The listing builds one solid part. Answer for the finished solid, in the listing's coordinates (mm). A direction names the side the tool comes from. Give positions to 0.01 mm unless a question says otherwise; leave off trailing zeros. Order: outer loops, then holes, each group sorted by start corner. A loop starts at its lowest first (then second) coordinate and runs counter-clockwise, first axis right, second up. Notation, with made-up numbers: (-26, -25.5) - (12, -25.5) arc R29 ccw to (12, 1.5) - close; hole circle Ø1 at (83.5, 89.5). An arc over 180 degrees is marked (long way). Answer in a Markdown table with one row per item. Add a question column.
Autodesk Inventor part; units mm, degrees
ref_plane "YZ Plane" through (0, 0, 0) normal (1, 0, 0) x (0, 1, 0)
ref_plane "XZ Plane" through (0, 0, 0) normal (0, 1, 0) x (-1, 0, 0)
ref_plane "XY Plane" through (0, 0, 0) normal (0, 0, 1) x (1, 0, 0)
sketch "Sketch1" plane through (0, 0, 0) normal (0, 0, 1) x (1, 0, 0)
  line L0 (0, 0) -> (50, 0)
  line L1 (50, 0) -> (50, -40)
  line L2 (50, -40) -> (0, -40)
  line L3 (0, -40) -> (0, 0)
  dimension "d0" = 50
  dimension "d1" = 40
extrude "Extrusion1" add sketch "Sketch1" along normal blind 60
shell "Shell1" thickness 1 outward yes removed faces 1 at (33.3333, 0, 20)
sketch "Sketch2" plane through (0, 0, 61) normal (0, 0, 1) x (1, 0, 0)
  circle A0 centre (9, -10) radius 7.5
  line L0 (51, 0) -> (-1, 0)
  line L1 (-1, 0) -> (-1, -41)
  point P0 (0, 0)
  dimension "d5" = 10
  dimension "d6" = 10
  dimension "d7" = 15
extrude "Extrusion2" cut sketch "Sketch2" against normal blind 60
properties part number "Part4 zaid"
(1) Find section D-D, the plane x = 28. Write down the section's boundary in (y, z).
(2) The mould has two halves that part along Y. Classify faces 3 (the face through (25, -40, 30)), 4 (the face through (1.507, -9.67, 60.507)), 5 (the face through (51, -20, 30)), 6 (the face through (25, -41, 30)): +Y half, -Y half, draft (parallel to the pull), parting line (faces both ways), or undercut.
(3) For faces 1 (the face through (50, -20, 30)), 2 (the face through (-0.2, 0, 29.9)), determine the directions among +Z, -Z, +X, -X, +Y, -Y from which every point of the face is accessible in a straight line to the end or side of a thin tool.
(4) Each of these flat-tipped pins is pushed along its axis until it touches: P1, Ø8, axis at x = 34.5, z = 47.5, coming from the +Y side; P2, Ø13.5, axis at x = 9, y = -10, coming from the +Z side. Where does it stop, or does it pass through?
(5) Straight lines are drawn through the part: line 1 (Y direction, x = 9, z = 60.65); line 2 (X direction, y = -36, z = 28.5); line 3 (Z direction, x = 24, y = -23). For each, find the intervals that lie inside material, in ascending order.
(6) Find section B-B, the plane y = -31. Write down the section's boundary in (x, z).
(7) Find section A-A, the plane x = 9. Write down the section's boundary in (y, z), plus the area to 3 significant figures.
(8) Find section C-C, the plane z = 12. Write down the section's boundary in (x, y), plus the area to 3 significant figures.
Answer key:
| question | item | result |
|---|---|---|
| 1 | outline | (-41, -1) - (0, -1) - (0, 0) - (-40, 0) - (-40, 60) - (0, 60) - (0, 61) - (-41, 61) - close |
| 2 | face 3 | +Y half |
| 2 | face 4 | undercut |
| 2 | face 5 | draft |
| 2 | face 6 | -Y half |
| 3 | face 1 | +Y |
| 3 | face 2 | +Z, -Z, +X, -X, +Y |
| 4 | P1 | y = -40 |
| 4 | P2 | z = 0 |
| 5 | line 1 | -41 to -17.5, -2.5 to 0 |
| 5 | line 2 | -1 to 0, 50 to 51 |
| 5 | line 3 | -1 to 0, 60 to 61 |
| 6 | outline | (-1, -1) - (51, -1) - (51, 61) - (-1, 61) - close; hole (0, 0) - (50, 0) - (50, 60) - (0, 60) - close |
| 7 | outline | (-41, -1) - (0, -1) - (0, 0) - (-40, 0) - (-40, 60) - (-17.5, 60) - (-17.5, 61) - (-41, 61) - close; (-2.5, 60) - (0, 60) - (0, 61) - (-2.5, 61) - close |
| 7 | area | 127 mm² |
| 8 | outline | (-1, -41) - (51, -41) - (51, 0) - (50, 0) - (50, -40) - (0, -40) - (0, 0) - (-1, 0) - close |
| 8 | area | 132 mm² |
